Check sheet for the drawn part. Datum: minimum x, y, z corner. Units: mm. A direction names the side the tool comes from. Round coordinates to 2 decimals unless told otherwise and drop trailing zeros. Write each loop counter-clockwise with the first axis right and the second up, starting at its lowest first coordinate (ties: lowest second). Pieces come first, ordered by that corner, then holes. Notation, with made-up numbers: (-13.75, 14) - (24.25, 14) arc R30 cw to (24.25, 42) - close; hole circle Ø2 at (35, 80). An arc over 180 degrees is marked (long way). Answer as a JSON object with one key per item and string values.
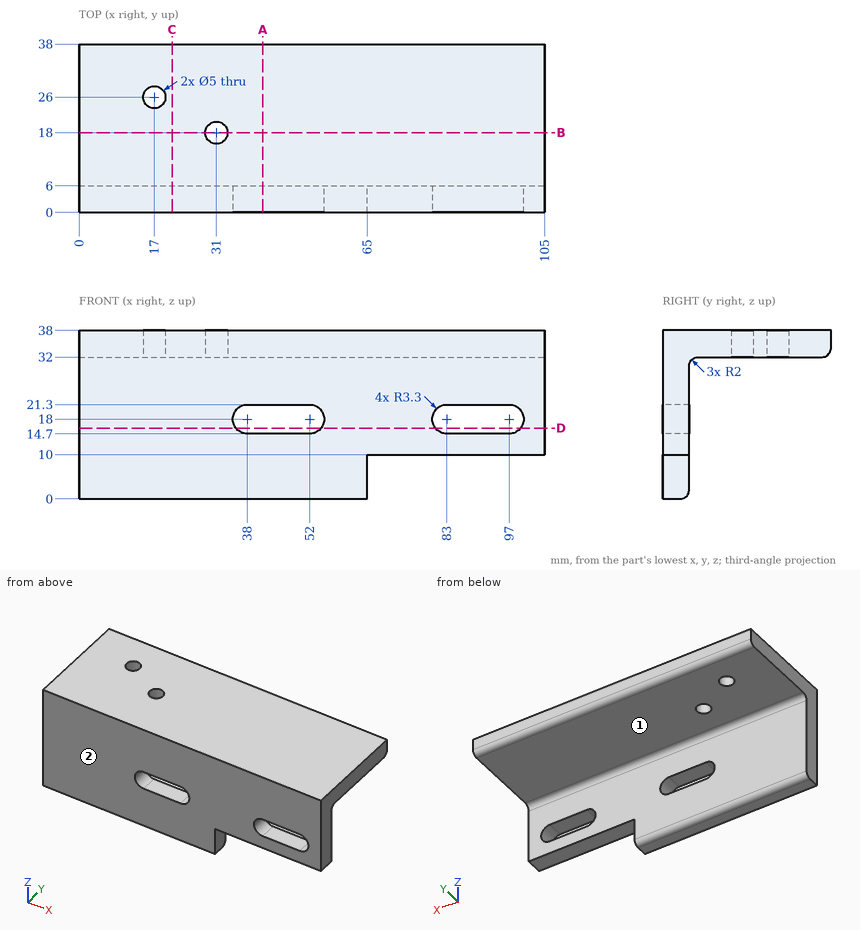
1. Cross-section at C-C (x = 21). Record the boundary of the cut face in (y, z), plus the area to 3 significant figures.
Completed:
{"outline": "(0, 0) - (4, 0) arc R2 ccw to (6, 2) - (6, 30) arc R2 cw to (8, 32) - (36, 32) arc R2 ccw to (38, 34) - (38, 38) - (0, 38) - close", "area": "419 mm^2"}
2. Cross-section at A-A (x = 41.5). Record the boundary of the cut face in (y, z), plus the area to 3 significant figures.
Completed:
{"outline": "(0, 0) - (4, 0) arc R2 ccw to (6, 2) - (6, 14.7) - (0, 14.7) - close; (0, 21.3) - (6, 21.3) - (6, 30) arc R2 cw to (8, 32) - (36, 32) arc R2 ccw to (38, 34) - (38, 38) - (0, 38) - close", "area": "380 mm^2"}
3. Go/stop test with flat-tipped pins: pin 1 (6.5 mm diameter, centred on x = 80.5, y = 2, fed in from -Z); pin 2 (3 mm diameter, centred on x = 19.5, z = 17, fed in from +Y); pin 3 (8.5 mm diameter, centred on x = 27.5, y = 15.5, fed in from -Z). Record where each tip stops, or that it passes through.
Completed:
{"pin 1": "stops at z = 10", "pin 2": "stops at y = 6", "pin 3": "stops at z = 32"}
4. Cross-section at B-B (y = 18). Record the boundary of the cut face in (x, z).
Completed:
{"outline": "(0, 32) - (28.5, 32) - (28.5, 38) - (0, 38) - close; (33.5, 32) - (105, 32) - (105, 38) - (33.5, 38) - close"}
5. Material ranges on probe 1 along Z at (x, y) = (68, 8.5); probe 2 along Y at (x, z) = (17, 34.8); probe 3 along Y at (x, z) = (5, 6), recorded low to high. Write a range as from..to.
Completed:
{"probe 1": "z = 32..38", "probe 2": "y = 0..23.5, 28.5..38", "probe 3": "y = 0..6"}
6. Cross-section at D-D (z = 16). Record the boundary of the cut face in (x, y).
Completed:
{"outline": "(0, 0) - (35.38, 0) - (35.38, 6) - (0, 6) - close; (54.62, 0) - (80.38, 0) - (80.38, 6) - (54.62, 6) - close; (99.62, 0) - (105, 0) - (105, 6) - (99.62, 6) - close"}
7. Access from +Z, -Z, +X, -X, +Y, -Y to the whole of each face (thin tool, end or side, straight path). Record for the marked faces 1 and 2.
Completed:
{"face 1": "-Z, +X, -X, +Y", "face 2": "+Z, -Z, +X, -X, -Y"}
